Autodesk Inventor part; units mm, degrees
ref_plane "YZ Plane" through (0, 0, 0) normal (1, 0, 0) x (0, 1, 0)
ref_plane "XZ Plane" through (0, 0, 0) normal (0, 1, 0) x (-1, 0, 0)
ref_plane "XY Plane" through (0, 0, 0) normal (0, 0, 1) x (1, 0, 0)
sketch "Sketch1" plane through (0, 0, 0) normal (0, 0, 1) x (1, 0, 0)
  line L0 (0, -120) -> (0, 155.2673)
  line L1 (-130, 0) -> (-130, 5)
  line L2 (-10, 5) -> (0, 5)
  line L3 (0, -74) -> (-9.8, -74)
  line L4 (-130, 5) -> (-120, 5)
  line L5 (-120.2, -74) -> (-129.8, -74)
  line L6 (-129.8, -69) -> (-129.8, -74)
  line L7 (0, 5) -> (-78.1654, 5)
  line L8 (-78.1654, 5) -> (-78.1654, -74)
  line L9 (-78.1654, -74) -> (0, -74)
  line L10 (0, -74) -> (0, 5)
  line L11 (-155.5538, 0) -> (-155.5538, 5)
  line L12 (-170.1, 0) -> (-170.1, 5)
  line L13 (-78.2654, -73) -> (-78.2654, -4)
  point P0 (0, 0)
  dimension "d36" = 0.1
extrude "Extrusion1" add sketch "Sketch1" along normal blind 6
sketch "Sketch2" plane through (0, 0, 6) normal (0, 0, 1) x (1, 0, 0)
  line L0 (-10, 0) -> (-10, 5)
  line L1 (0, 5) -> (-78.1654, 5)
  line L2 (-20, 0) -> (-10, 0)
  line L3 (-20, 5) -> (-20, 0)
  line L4 (-9.9, 5) -> (-9.9, 0)
  line L5 (-20.1, 0) -> (-20.1, 5)
  line L6 (-10, 0) -> (-9.9, 0)
  line L7 (-20, 0) -> (-20.1, 0)
  point P0 (-130, 5)
extrude "Extrusion2" cut sketch "Sketch2" against normal blind 6
sketch "Sketch3" plane through (-20.1, 0, 6) normal (0, 1, 0) x (1, 0, 0)
  circle A0 centre (5.1, 3) radius 1.5
  point P0 (20.1, 6)
hole "Hole1" at (-15, 0, 3) direction (0, -1, 0) diameter 2.8 depth 20
pattern_linear "Rectangular Pattern2" count 9 spacing 20 along (-1, 0, 0) of "Extrusion2", "Hole1"
ref_plane "Work Plane1" through (-20.1, -34.5, 6) normal (0, 1, 0) x (1, 0, 0)
mirror "Mirror1" about plane through (-20.1, -34.5, 6) normal (0, 1, 0) of "Extrusion2", "Hole1", "Rectangular Pattern2"
properties part number "00_Baseplate_Simmo_side5"
Geometry: final body of the model. Coordinates: model frame, mm. A direction names the side the tool comes from. Coordinates: 2 decimals unless noted, no trailing zeros. Order: outer loops, then holes, each group sorted by start corner. A loop starts at its lowest first (then second) coordinate and runs counter-clockwise, first axis right, second up.
(1) Draft query along X for faces 1 (the face through (-35, -20, 3)), 2 (the face through (-45, -74, 3)), 3 (the face through (-69.9, -71, 3)), 4 (the face through (-16.18, -10.14, 3.75)). Return one class per face: pulls with the +X half, pulls with the -X half, needs draft (parallel to the pull), parting line crosses it, or undercut.
(2) Section query B-B (x = -15). Return the cut outline in (y, z), plus the area to 3 significant figures.
(3) First-contact query: pin 1 (1.8 mm diameter, centred on x = -55.5, z = 1.5, fed in from +Y); pin 2 (2 mm diameter, centred on x = -15, z = 3, fed in from -Y); pin 3 (2.5 mm diameter, centred on y = 2.5, z = 4.5, fed in from -X). Flat tips, straight axial feed; report the tip coordinate or a pass-through.
(4) Section query A-A (y = -12). Return the cut outline in (x, z).
(5) Material intervals for probe 1 along X at (y, z) = (-60, 3); probe 2 along Z at (x, y) = (-15, -53); probe 3 along Y at (x, z) = (-53, 5.1), sorted ascending.
(6) Access query for faces 5 (the face through (-20.1, -72, 3)), 6 (the face through (-73, 0, 3)), 7 (the face through (-56.2, 0, 4.4)). Directions: +Z, -Z, +X, -X, +Y, -Y. A direction counts if a zero-diameter tool reaches every point of the face in a straight line with its end or side. Return the directions, or none.
Solution:
1. face 1: undercut
1. face 2: needs draft
1. face 3: pulls with the -X half
1. face 4: undercut
2. outline: (-69, 0) - (0, 0) - (0, 1.6) - (-20, 1.6) - (-20, 4.4) - (0, 4.4) - (0, 6) - (-69, 6) - (-69, 4.4) - (-49, 4.4) - (-49, 1.6) - (-69, 1.6) - close
2. area: 302 mm2
3. pin 1: stops at y = 0
3. pin 2: stops at y = -49
3. pin 3: stops at x = -69.9
4. outline: (-78.17, 0) - (0, 0) - (0, 6) - (-78.17, 6) - close; hole circle Ø2.8 at (-75, 3); hole circle Ø2.8 at (-55, 3); hole circle Ø2.8 at (-35, 3); hole circle Ø2.8 at (-15, 3)
5. probe 1: x = -78.17 to -76.4, -73.6 to -56.4, -53.6 to -36.4, -33.6 to -16.4, -13.6 to 0
5. probe 2: z = 0 to 1.6, 4.4 to 6
5. probe 3: y = -69 to 0
6. face 5: +Z, -Z, -Y
6. face 6: +Z, -Z, -X, +Y
6. face 7: +Z, -Z, +Y
